```python
from build123d import *

# Parameters (mm, degrees)
SKETCH1_R           = 25.4
BOSS_EXTRUDE1_DEPTH = 6.35


with BuildPart() as part:
    # Sketch1 → Boss-Extrude1 (new body)
    with BuildSketch(Plane.XY):
        with Locations((-8.514653882, 2.430473335)):
            Circle(SKETCH1_R)
        with BuildLine():
            Line((-2.121320344, 1.75), (2.121320344, 1.75))
            ThreePointArc((2.121320344, 1.75), (2.75, 0), (2.121320344, -1.75))
            Line((2.121320344, -1.75), (-2.121320344, -1.75))
            ThreePointArc((-2.121320344, -1.75), (-2.75, 0), (-2.121320344, 1.75))
        make_face(mode=Mode.SUBTRACT)
    extrude(amount=BOSS_EXTRUDE1_DEPTH)


solid = part.part
```
Geometry check sheet. Reference: the model listing, model coordinates, mm. A direction names the side the tool comes from. Coordinates: 2 decimals unless noted, no trailing zeros. Order: outer loops, then holes, each group sorted by start corner. A loop starts at its lowest first (then second) coordinate and runs counter-clockwise, first axis right, second up. Notation, with made-up numbers: (58, 77) - (82, 77) arc R30 ccw to (82, 105) - close; hole circle Ø4 at (-35, -11.75). An arc over 180 degrees is marked (long way). Answer as a JSON object with one key per item and string values. Group by question number.
Item 1: Depth check by flat-ended pin: pin 1 Ø1 at (y, z) = (19.5, 1) entering from +X; pin 2 Ø3.5 at (x, z) = (-0.5, 2.5) entering from +Y; pin 3 Ø1 at (y, z) = (21.5, 0.5) entering from +X. Enter the tip coordinate at first touch or a pass-through.
Item 2: Tool access check on faces 1 (the face through (0, -1.75, 3)), 2 (the face through (-9, 3, 6.35)). Record the directions out of +Z, -Z, +X, -X, +Y, -Y that give a thin tool (end or side, any length) a straight path to the whole face; none if there is none.
Item 3: Scan lines: probe 1 along Y at (x, z) = (2.5, 3.5); probe 2 along Y at (x, z) = (-11.5, 3.5); probe 3 along X at (y, z) = (17, 4.75). Record each from-to range of solid material in increasing order.
Item 4: Sectioned sample at C-C, the plane z = 4. Record the cut outline in (x, y), and give its area (3 significant figures).
Item 5: Sectioned sample at D-D, the plane x = 4.5. Record the cut outline in (y, z).
Item 6: Draft check along Y on faces 3 (the face through (-9, 3, 0)), 4 (the face through (15.7, 10.1, 3.1)), 5 (the face through (0, 1.75, 3)). Enter one of: +Y half, -Y half, draft (parallel to the pull), parting line (faces both ways), or undercut.
Item 7: Sectioned sample at A-A, the plane x = -1.5. Record the cut outline in (y, z), and give its area (3 significant figures).
Item 8: Sectioned sample at B-B, the plane y = 0. Record the cut outline in (x, z), and give its area (3 significant figures).
Resolved:
{
 "1": {"pin 1": "x = 10.74", "pin 2": "y = 27.05", "pin 3": "x = 8.82"},
 "2": {"face 1": "+Z, -Z", "face 2": "+Z, +X, -X, +Y, -Y"},
 "3": {"probe 1": "-20.46 to -1.15, 1.15 to 25.32", "probe 2": "-22.79 to 27.65", "probe 3": "-29.32 to 12.29"},
 "4": {"outline": "circle Ø50.8 at (-8.51, 2.43); hole (-2.12, -1.75) - (2.12, -1.75) arc R2.75 ccw to (2.12, 1.75) - (-2.12, 1.75) arc R2.75 ccw to start", "area": "2,010 mm^2"},
 "5": {"outline": "(-19.38, 0) - (24.24, 0) - (24.24, 6.35) - (-19.38, 6.35) - close"},
 "6": {"face 3": "draft", "face 4": "parting line", "face 5": "undercut"},
 "7": {"outline": "(-21.98, 0) - (-1.75, 0) - (-1.75, 6.35) - (-21.98, 6.35) - close; (1.75, 0) - (26.84, 0) - (26.84, 6.35) - (1.75, 6.35) - close", "area": "288 mm^2"},
 "8": {"outline": "(-33.8, 0) - (-2.75, 0) - (-2.75, 6.35) - (-33.8, 6.35) - close; (2.75, 0) - (16.77, 0) - (16.77, 6.35) - (2.75, 6.35) - close", "area": "286 mm^2"}
}
